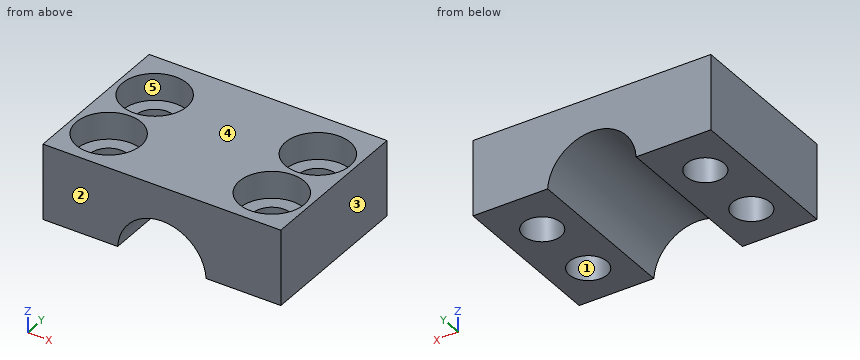
```python
from build123d import *

# Parameters (mm, degrees)
PAD008_DEPTH    = 15
SKETCH018_R     = 1.75
POCKET008_DEPTH = 7.001
SKETCH019_R     = 3
POCKET009_DEPTH = 2.5


with BuildPart() as part:
    # Sketch017 (on Face1 of ReferencePocket007) → Pad008 (new body)
    with BuildSketch(Plane(origin=(0, -9.8, 0), x_dir=(-1, 0, 0), z_dir=(0, 1, 0))):
        with BuildLine():
            ThreePointArc((15.0923709509, 0.25), (11, 4.1), (6.9076290491, 0.25))
            Line((6.9076290491, 0.25), (0, 0.25))
            Line((0, 0.25), (0, 7.25))
            Line((0, 7.25), (22, 7.25))
            Line((22, 7.25), (22, 0.25))
            Line((15.0923709509, 0.25), (22, 0.25))
        make_face()
    extrude(amount=-PAD008_DEPTH)

    # Sketch018 (on Face6 of Pad008) → Pocket008 (cut, through all)
    with BuildSketch(Plane(origin=(0, 0, 0.25), x_dir=(1, 0, 0), z_dir=(0, 0, -1))):
        with Locations((-18.5461854755, 14.3)):
            Circle(SKETCH018_R)
        with Locations((-18.5461854755, 20.8)):
            Circle(SKETCH018_R)
        with Locations((-3.4538145245, 20.8)):
            Circle(SKETCH018_R)
        with Locations((-3.4538145245, 14.3)):
            Circle(SKETCH018_R)
    extrude(amount=-POCKET008_DEPTH, mode=Mode.SUBTRACT)

    # Sketch019 (on Face12 of Pocket008) → Pocket009 (cut)
    with BuildSketch(Plane.XY.offset(7.25)):
        with Locations((-18.5461854755, -14.3)):
            Circle(SKETCH019_R)
        with Locations((-18.5461854755, -20.8)):
            Circle(SKETCH019_R)
        with Locations((-3.4538145245, -20.8)):
            Circle(SKETCH019_R)
        with Locations((-3.4538145245, -14.3)):
            Circle(SKETCH019_R)
    extrude(amount=-POCKET009_DEPTH, mode=Mode.SUBTRACT)


solid = part.part
```
Work out the finished part from the listing and answer in its coordinate system (mm). Face numbers are marked on the shaded views. A direction names the side the tool comes from. Coordinates: 2 decimals unless noted, no trailing zeros. Loops run counter-clockwise (first coordinate to the right, second up) from the corner with the lowest first, then second, coordinate; pieces in that order, holes last. Notation, with made-up numbers: M -6,33 L 6,33 A4 ccw 6,39 Z; hole C -15.75,18 d6. An arc over 180 degrees is marked long. Use CSV: the item, a comma, the result in double quotes. Start each with the question number.
(1) Given pin 1 Ø3 at (x, y) = (-3.45, -14.3) entering from -Z; pin 2 Ø3 at (x, y) = (-19.5, -14.5) entering from +Z, each flat-ended and moving along its own axis, determine where each tip first touches the part or whether it passes through.
(2) Consider line 1 (Y direction, x = -19.5, z = 6.25); line 2 (Y direction, x = -4.25, z = 4); line 3 (X direction, y = -14, z = 0.75). Determine where each line is inside the solid, lowest interval first.
(3) For the marked faces 4 and 5, determine the directions among +Z, -Z, +X, -X, +Y, -Y from which every point of the face is accessible in a straight line to the end or side of a thin tool.
(4) For a pull along Y with two mould halves and no side action, classify the marked faces 1, 2 and 3 as +Y half, -Y half, draft (parallel to the pull), parting line (faces both ways), or undercut.
(5) Find section B-B, the plane z = 1.75. Give the vertices of the cut face in (x, y).
(6) Find section A-A, the plane y = -20.8. Give the vertices of the cut face in (x, z), then the cut area to 3 significant figures.
(7) Find section C-C, the plane x = -19.5. Give the vertices of the cut face in (y, z), then the cut area to 3 significant figures.
(8) Find section D-D, the plane z = 6.5. Give the vertices of the cut face in (x, y).
Recorded:
1,pin 1,"passes through"
1,pin 2,"stops at z = 4.75"
2,line 1,"y = -24.8 to -23.64, -17.96 to -17.14, -11.46 to -9.8"
2,line 2,"y = -24.8 to -22.36, -19.24 to -15.86, -12.74 to -9.8"
2,line 3,"x = -22 to -20.27, -16.82 to -15.03, -6.97 to -5.18, -1.73 to 0"
3,face 4,"+Z, +X, -X, +Y, -Y"
3,face 5,"+Z"
4,face 1,"undercut"
4,face 2,"-Y half"
4,face 3,"draft"
5,outline,"M -22,-24.8 L -14.71,-24.8 L -14.71,-9.8 L -22,-9.8 Z; M -7.29,-24.8 L 0,-24.8 L 0,-9.8 L -7.29,-9.8 Z; hole C -18.55,-20.8 d3.5; hole C -18.55,-14.3 d3.5; hole C -3.45,-20.8 d3.5; hole C -3.45,-14.3 d3.5"
6,outline,"M -22,0.25 L -20.3,0.25 L -20.3,4.75 L -21.55,4.75 L -21.55,7.25 L -22,7.25 Z; M -16.8,0.25 L -15.09,0.25 A4.1 cw -6.91,0.25 L -5.2,0.25 L -5.2,4.75 L -6.45,4.75 L -6.45,7.25 L -15.55,7.25 L -15.55,4.75 L -16.8,4.75 Z; M -1.7,0.25 L 0,0.25 L 0,7.25 L -0.45,7.25 L -0.45,4.75 L -1.7,4.75 Z"
6,area,"68.1 mm^2"
7,outline,"M -24.8,0.25 L -22.27,0.25 L -22.27,4.75 L -23.64,4.75 L -23.64,7.25 L -24.8,7.25 Z; M -19.33,0.25 L -15.77,0.25 L -15.77,4.75 L -17.14,4.75 L -17.14,7.25 L -17.96,7.25 L -17.96,4.75 L -19.33,4.75 Z; M -12.83,0.25 L -9.8,0.25 L -9.8,7.25 L -11.46,7.25 L -11.46,4.75 L -12.83,4.75 Z"
7,area,"50.1 mm^2"
8,outline,"M -22,-24.8 L 0,-24.8 L 0,-9.8 L -22,-9.8 Z; hole C -18.55,-20.8 d6; hole C -18.55,-14.3 d6; hole C -3.45,-20.8 d6; hole C -3.45,-14.3 d6"
